Design review of the part built by this model. Coordinates are the model's own, in mm. A direction names the side the tool comes from. Coordinates: 2 decimals unless noted, no trailing zeros. Write each loop counter-clockwise with the first axis right and the second up, starting at its lowest first coordinate (ties: lowest second). Pieces come first, ordered by that corner, then holes. Notation, with made-up numbers: M -34,-23 L -19,-23 A32 ccw -19,13 Z; hole C 15.5,47 d7. An arc over 180 degrees is marked long. Return JSON: item names as keys, results as strings. Group by question number.
```python
from build123d import *

# Parameters (mm, degrees)
EXTRUDE_1_DEPTH          = 6
EXTRUDE_1_DEPTH_BACK     = 6
CUT_EXTRUDE_1_DEPTH      = 3
CUT_EXTRUDE_1_DEPTH_BACK = 3
SKETCH_4_R               = 4


with BuildPart() as part:
    # Sketch 1 → Extrude 1 (new, two sides: drawn at the far end of the back side and taken through both)
    with BuildSketch(Plane.XY.offset(-EXTRUDE_1_DEPTH_BACK)):
        with BuildLine():
            Line((0, -8), (27.5, -8))
            ThreePointArc((27.5, -8), (35.5, 0), (27.5, 8))
            Line((27.5, 8), (0, 8))
            ThreePointArc((0, 8), (-8, 0), (0, -8))
        make_face()
    extrude(amount=EXTRUDE_1_DEPTH + EXTRUDE_1_DEPTH_BACK)

    # Sketch 2 → Revolve 1 (revolve)
    with BuildSketch(Plane(origin=(0, 0, 0), x_dir=(0, 0, -1), z_dir=(1, 0, 0)), mode=Mode.PRIVATE) as revolve_1_sk:
        with BuildLine():
            Line((-6, 4.82182538), (-6, 4))
            Line((-6, 4), (6, 4))
            Line((6, 4), (6, 4.5))
            Line((6, 4.5), (7, 4.5))
            Line((7, 4.5), (7, 0))
            Line((7, 0), (-7.5, 0))
            ThreePointArc((-7.5, 0), (-7.11634154, 2.524876235), (-6, 4.82182538))
        make_face()
    revolve(revolve_1_sk.sketch.rotate(Axis((0, 0, -7), (0, 0, 1)), 180), axis=Axis((0, 0, -7), (0, 0, 1)))

    # Sketch 3 → Revolve 2 (revolve)
    with BuildSketch(Plane(origin=(27.5, 0, 0), x_dir=(0, 0, -1), z_dir=(1, 0, 0)), mode=Mode.PRIVATE) as revolve_2_sk:
        with BuildLine():
            Line((-6, 4.82182538), (-6, 4))
            Line((-6, 4), (6, 4))
            Line((6, 4), (6, 4.5))
            Line((6, 4.5), (7, 4.5))
            Line((7, 4.5), (7, 0))
            Line((7, 0), (-7.5, 0))
            ThreePointArc((-7.5, 0), (-7.11634154, 2.524876235), (-6, 4.82182538))
        make_face()
    revolve(revolve_2_sk.sketch.rotate(Axis((27.5, 0, -7), (0, 0, 1)), 180), axis=Axis((27.5, 0, -7), (0, 0, 1)))

    # Sketch 4 → Cut-Extrude 1 (cut, two sides: drawn at the far end of the back side and taken through both)
    with BuildSketch(Plane.XY.offset(-CUT_EXTRUDE_1_DEPTH_BACK)):
        with BuildLine():
            Line((0, -8), (27.5, -8))
            ThreePointArc((27.5, -8), (35.5, 0), (27.5, 8))
            Line((27.5, 8), (0, 8))
            ThreePointArc((0, 8), (-8, 0), (0, -8))
        make_face()
        with Locations((27.5, 0)):
            Circle(SKETCH_4_R, mode=Mode.SUBTRACT)
        Circle(SKETCH_4_R, mode=Mode.SUBTRACT)
    extrude(amount=CUT_EXTRUDE_1_DEPTH + CUT_EXTRUDE_1_DEPTH_BACK, mode=Mode.SUBTRACT)


solid = part.part
```
Item 1: Add section C-C (y = 0). Write out the cut boundary in (x, z), plus the area to 3 significant figures.
Item 2: Machinability: for faces 1 (the cylindrical face through (3.04, 3.32, -6.51)), 2 (the cylindrical face through (-0.867, -3.905, -0.042)), 3 (the flat face through (13, 0, 6)), which of the approach directions +Z, -Z, +X, -X, +Y, -Y give a long, thin tool a straight path to every point of the face, cutting with its end or side? Answer none if there is none.
Item 3: For line 1 (Z direction, x = 15.5, y = -3.25); line 2 (X direction, y = -2.5, z = -2); line 3 (X direction, y = -0.25, z = 2.75), list the stretches that pass through material, from the lowest coordinate up.
Item 4: Add section A-A (x = 17). Write out the cut boundary in (y, z).
Item 5: The part is to be moulded in two halves that separate along X. For faces 4 (the flat face through (13, 0, 3)), 5 (the cylindrical face through (35.498, -0.176, -4.521)), 6 (the flat face through (14, -8, 4)), 7 (the cylindrical face through (-8, 0, 4)), say which applies: pulls with the +X half, pulls with the -X half, needs draft (parallel to the pull), parting line crosses it, or undercut.
Item 6: Add section D-D (z = -0.25). Write out the cut boundary in (x, y), plus the area to 3 significant figures.
Item 7: For pin 1 (4 mm diameter, centred on y = 5, z = 4, fed in from -X); pin 2 (8 mm diameter, centred on y = 3.5, z = -2.5, fed in from -X); pin 3 (1 mm diameter, centred on y = 2.5, z = 4.5, fed in from +X); pin 4 (1.5 mm diameter, centred on x = 30, y = -4.5, fed in from +Z), all flat-tipped, find the tip position at first contact; note any pin that passes through.
Item 8: Add section B-B (y = 7). Write out the cut boundary in (x, z), plus the area to 3 significant figures.
Geometry check:
{
 "1": {"outline": "M -8,-6 L -4.5,-6 L -4.5,-7 L 4.5,-7 L 4.5,-6 L 23,-6 L 23,-7 L 32,-7 L 32,-6 L 35.5,-6 L 35.5,-3 L 31.5,-3 L 31.5,3 L 35.5,3 L 35.5,6 L 32.32,6 A8.5 ccw 22.68,6 L 4.82,6 A8.5 ccw -4.82,6 L -8,6 L -8,3 L -4,3 L -4,-3 L -8,-3 Z; hole M 4,-3 L 23.5,-3 L 23.5,3 L 4,3 Z", "area": "395 mm^2"},
 "2": {"face 1": "-Z", "face 2": "none", "face 3": "+Z"},
 "3": {"line 1": "-6 to -3, 3 to 6", "line 2": "-3.12 to 3.12, 24.38 to 30.62", "line 3": "-3.99 to 3.99, 23.51 to 31.49"},
 "4": {"outline": "M -8,-6 L 8,-6 L 8,-3 L -8,-3 Z; M -8,3 L 8,3 L 8,6 L -8,6 Z"},
 "5": {"face 4": "undercut", "face 5": "pulls with the +X half", "face 6": "needs draft", "face 7": "pulls with the -X half"},
 "6": {"outline": "C 0,0 d8; C 27.5,0 d8", "area": "101 mm^2"},
 "7": {"pin 1": "x = -7.42", "pin 2": "x = -8", "pin 3": "x = 35.25", "pin 4": "z = 6.27"},
 "8": {"outline": "M -3.87,-6 L 31.37,-6 L 31.37,-3 L -3.87,-3 Z; M -3.87,3 L 31.37,3 L 31.37,6 L -3.87,6 Z", "area": "211 mm^2"}
}
